from build123d import *

# Parameters (mm, degrees)
SKETCH_1_W                = 30
SKETCH_1_H                = 20
SKETCH_3_W                = 30
SKETCH_3_H                = 10
EXTRUDE_2_DEPTH           = 10
SKETCH_4_W                = 10
SKETCH_4_H                = 10
CUT_EXTRUDE_1_DEPTH       = 15
CUT_EXTRUDE_2_DEPTH       = 15
SKETCH_6_R                = 1.5
CUT_EXTRUDE_3_DEPTH       = 15
SKETCH_8_W                = 6
SKETCH_8_H                = 15
SKETCH_12_W               = 20
SKETCH_12_H               = 110
EXTRUDE_3_DEPTH           = 15
SKETCH_14_W               = 27
SKETCH_14_H               = 53
SKETCH_14_W_2             = 32.56993007
SKETCH_14_H_2             = 48
CUT_EXTRUDE_6_DEPTH       = 17
SKETCH_18_W               = 14.5
SKETCH_18_H               = 20
CUT_EXTRUDE_7_DEPTH       = 3
SKETCH_19_W               = 13.260290085
SKETCH_19_H               = 2.030039981
CUT_EXTRUDE_8_DEPTH       = 5
CUT_EXTRUDE_START         = 96.160609199
CUT_EXTRUDE_9_OUTLINE_W   = 4.260290085
CUT_EXTRUDE_9_OUTLINE_H   = 12
CUT_EXTRUDE_9_OUTLINE_W_2 = 3
CUT_EXTRUDE_9_DEPTH       = 2.030039981


# Read off the part's stored shape, not the designer's step: 切除-拉伸9
with BuildPart() as part:
    # Sweep 1: sweep along a path in 草图2
    with BuildLine(Plane(origin=(-2.57, 0, 0), x_dir=(0, 0, -1), z_dir=(1, 0, 0))) as sweep_1_path:
        Line((-5.367132867, 0), (-5.367132867, 110))
        Line((-5.367132867, 110), (-30.540121802, 140))
    # 草图1 → Sweep 1 (sweep)
    with BuildSketch(Plane(origin=(0, 0, 0), x_dir=(1, 0, 0), z_dir=(0, 1, 0))):
        with Locations((-2.56993007, -5.367132867)):
            Rectangle(SKETCH_1_W, SKETCH_1_H)
    sweep(path=sweep_1_path.line, transition=Transition.RIGHT)

    # 草图3 → 凸台-拉伸2 (add)
    with BuildSketch(Plane.XZ):
        with Locations((-2.56993007, 0.367132867)):
            Rectangle(SKETCH_3_W, SKETCH_3_H)
    extrude(amount=EXTRUDE_2_DEPTH)

    # 草图4 → 切除-拉伸1 (cut)
    with BuildSketch(Plane(origin=(12.43006993, 0, 0), x_dir=(0, 0, -1), z_dir=(1, 0, 0))):
        with Locations((-0.367132867, -5)):
            Rectangle(SKETCH_4_W, SKETCH_4_H)
    extrude(amount=-CUT_EXTRUDE_1_DEPTH, mode=Mode.SUBTRACT)

    # 草图5 → 切除-拉伸2 (cut)
    with BuildSketch(Plane.ZY.offset(17.56993007)):
        with BuildLine():
            Line((5.367132867, -10), (0.367132867, -10))
            ThreePointArc((0.367132867, -10), (3.902666773, -8.535533906), (5.367132867, -5))
            Line((5.367132867, -5), (5.367132867, -10))
        make_face()
    extrude(amount=-CUT_EXTRUDE_2_DEPTH, mode=Mode.SUBTRACT)

    # 草图6 → 切除-拉伸3 (cut)
    with BuildSketch(Plane.ZY.offset(17.56993007)):
        with Locations((0.367132867, -5)):
            Circle(SKETCH_6_R)
    extrude(amount=-CUT_EXTRUDE_3_DEPTH, mode=Mode.SUBTRACT)

    # Sweep 1 2: sweep along a path in 草图10
    with BuildLine(Plane(origin=(6.43006993, 0, 0), x_dir=(0, 0, -1), z_dir=(1, 0, 0))) as sweep_1_2_path:
        Line((-32.45523291, 138.393030976), (-7.867132867, 109.090074414))
        Line((-7.867132867, 109.090074414), (-7.867132867, 0))
    # 草图8 → Sweep 1 2 (sweep, cut)
    with BuildSketch(Plane(origin=(0, 97.193446801, 81.554985364), x_dir=(1, 0, 0), z_dir=(0, 0.7660444431189773, 0.6427876096865403))):
        with Locations((6.43006993, 64.095174757)):
            Rectangle(SKETCH_8_W, SKETCH_8_H)
    sweep(path=sweep_1_2_path.line, transition=Transition.RIGHT, mode=Mode.SUBTRACT)

    # 草图12 → 凸台-拉伸3 (add)
    with BuildSketch(Plane.ZY.offset(17.56993007)):
        with Locations((5.367132867, 56)):
            Rectangle(SKETCH_12_W, SKETCH_12_H)
    extrude(amount=EXTRUDE_3_DEPTH)

    # 草图14 → 切除-拉伸6 (cut)
    with BuildSketch(Plane(origin=(0, 0, -4.632867133), x_dir=(-1, 0, 0), z_dir=(0, 0, -1))):
        with Locations((19.06993007, 81.5)):
            Rectangle(SKETCH_14_W, SKETCH_14_H)
        with Locations((16.284965035, 28.17035924)):
            Rectangle(SKETCH_14_W_2, SKETCH_14_H_2)
    extrude(amount=-CUT_EXTRUDE_6_DEPTH, mode=Mode.SUBTRACT)

    # 草图18 → 切除-拉伸7 (cut)
    with BuildSketch(Plane(origin=(0, 0, -4.632867133), x_dir=(-1, 0, 0), z_dir=(0, 0, -1))):
        with Locations((-5.18006993, 90.294394936)):
            Rectangle(SKETCH_18_W, SKETCH_18_H)
    extrude(amount=-CUT_EXTRUDE_7_DEPTH, mode=Mode.SUBTRACT)

    # 草图19 → 切除-拉伸8 (cut)
    with BuildSketch(Plane(origin=(0, 0, -1.632867133), x_dir=(-1, 0, 0), z_dir=(0, 0, -1))):
        with Locations((-5.799924888, 97.17562919)):
            Rectangle(SKETCH_19_W, SKETCH_19_H)
    extrude(amount=-CUT_EXTRUDE_8_DEPTH, mode=Mode.SUBTRACT)

    # 切除-拉伸9 outline → 切除-拉伸9 (cut)
    with BuildSketch(Plane(origin=(0, 0, 0), x_dir=(1, 0, 0), z_dir=(0, 1, 0)).offset(CUT_EXTRUDE_START)):
        with Locations((1.299924888, -9.367132867)):
            Rectangle(CUT_EXTRUDE_9_OUTLINE_W, CUT_EXTRUDE_9_OUTLINE_H)
        with Locations((10.93006993, -9.367132867)):
            Rectangle(CUT_EXTRUDE_9_OUTLINE_W_2, CUT_EXTRUDE_9_OUTLINE_H)
    extrude(amount=CUT_EXTRUDE_9_DEPTH, mode=Mode.SUBTRACT)


solid = part.part
Geometry: final body of the model. Coordinates: model frame, mm. A direction names the side the tool comes from. Give positions to 0.01 mm unless a question says otherwise; leave off trailing zeros. Loops run counter-clockwise (first coordinate to the right, second up) from the corner with the lowest first, then second, coordinate; pieces in that order, holes last. Notation, with made-up numbers: (12.25, 33.5) -> (37.25, 33.5) arc R23 cw to (37.25, 72.5) -> close; hole circle Ø3 at (58.5, 3.25). An arc over 180 degrees is marked (long way). Put each result on its own line as item: value.
1. Cut plane B-B (x = -27). Return the cut outline in (y, z), plus the area to 3 significant figures.
Taken from the geometry:
outline: (1, -4.63) -> (4.17, -4.63) -> (4.17, 12.37) -> (52.17, 12.37) -> (52.17, -4.63) -> (55, -4.63) -> (55, 12.37) -> (108, 12.37) -> (108, -4.63) -> (111, -4.63) -> (111, 15.37) -> (1, 15.37) -> close
area: 483 mm2
2. Pin query (flat end, axial travel): P1, Ø6, axis at x = -10, y = 46.5, coming from the +Z side; P2, Ø18.5, axis at x = -13.5, z = 0.5, coming from the +Y side; P3, Ø1, axis at x = -13, y = 16, coming from the -Z side. Return the tip coordinate at first contact, or that it passes through.
Taken from the geometry:
P1: stops at z = 15.37
P2: stops at y = 130.78
P3: stops at z = 12.37
3. Cut plane A-A (z = 7.5). Return the cut outline in (x, y).
Taken from the geometry:
outline: (-32.57, 1) -> (-17.57, 1) -> (-17.57, 0) -> (3.43, 0) -> (3.43, 96.16) -> (-0.83, 96.16) -> (-0.83, 98.19) -> (3.43, 98.19) -> (3.43, 120.32) -> (9.43, 120.32) -> (9.43, 98.19) -> (12.43, 98.19) -> (12.43, 128.1) -> (-17.57, 128.1) -> (-17.57, 111) -> (-32.57, 111) -> (-32.57, 108) -> (-5.57, 108) -> (-5.57, 55) -> (-32.57, 55) -> (-32.57, 52.17) -> (0, 52.17) -> (0, 4.17) -> (-32.57, 4.17) -> close; (9.43, 0) -> (12.43, 0) -> (12.43, 96.16) -> (9.43, 96.16) -> close
4. Ray query, line 1 along Y through (x, z) = (-21, 11); line 2 along X through (y, z) = (82, 9.5); line 3 along X through (y, z) = (52.5, 6). Return the intervals inside material, ascending. Write a range as [from, to].
Taken from the geometry:
line 1: y = [1, 4.17], [52.17, 55], [108, 111]
line 2: x = [-5.57, 3.43], [9.43, 12.43]
line 3: x = [-32.57, 3.43], [9.43, 12.43]
5. Pull-direction query (X, two-part tool) for faces 5 (the flat face through (-5.57, 81, 4)), 6 (the flat face through (3, 98.191, 7)), 7 (the flat face through (3.43, 50, 10)); classes: released by +X, released by -X, zero draft, split by the parting line, or undercut.
Taken from the geometry:
face 5: released by -X
face 6: zero draft
face 7: undercut
6. Cut plane D-D (z = 14). Return the cut outline in (x, y), plus the area to 3 significant figures.
Taken from the geometry:
outline: (-32.57, 1) -> (-17.57, 1) -> (-17.57, 0) -> (3.43, 0) -> (3.43, 96.16) -> (-0.83, 96.16) -> (-0.83, 98.19) -> (3.43, 98.19) -> (3.43, 128.07) -> (9.43, 128.07) -> (9.43, 98.19) -> (12.43, 98.19) -> (12.43, 135.85) -> (-17.57, 135.85) -> (-17.57, 111) -> (-32.57, 111) -> close; (9.43, 0) -> (12.43, 0) -> (12.43, 96.16) -> (9.43, 96.16) -> close
area: 4,940 mm2
7. Cut plane C-C (y = 40.5). Return the cut outline in (x, z).
Taken from the geometry:
outline: (-32.57, 12.37) -> (0, 12.37) -> (0, -4.63) -> (12.43, -4.63) -> (12.43, 15.37) -> (9.43, 15.37) -> (9.43, 0.37) -> (3.43, 0.37) -> (3.43, 15.37) -> (-32.57, 15.37) -> close
8. Set-up query: faces 1 (the flat face through (-19, 82, 12.367)), 2 (the flat face through (11, 102, 15.367)), 3 (the flat face through (5, 90, -1.633)), 4 (the flat face through (6, 47, 0.367)). Return all of +Z, -Z, +X, -X, +Y, -Y with unobstructed straight access to the full face (end or side cutting, diameter ignored); none if empty.
Taken from the geometry:
face 1: -Z, -X
face 2: +Z, +X, -X, -Y
face 3: -Z, +X
face 4: +Z, -Y
